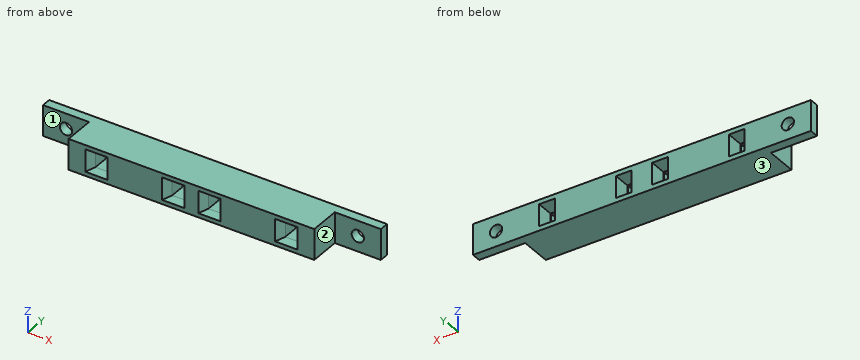
```python
from build123d import *

# Parameters (mm, degrees)
SKETCH1_W           = 80
SKETCH1_H           = 10
BOSS_EXTRUDE1_DEPTH = 10
SKETCH2_W           = 4.7
SKETCH2_H           = 6.7
CUT_EXTRUDE1_DEPTH  = 7
SKETCH3_W           = 4.7
SKETCH3_H           = 6.7
SKETCH4_W           = 7.3
SKETCH4_H           = 7.3
SKETCH5_W           = 4.7
SKETCH5_H           = 6.7
SKETCH6_W           = 7.3
SKETCH6_H           = 7.3
SKETCH8_W           = 4.7
SKETCH8_H           = 6.7
SKETCH9_W           = 7.3
SKETCH9_H           = 7.3
SKETCH10_W          = 4.7
SKETCH10_H          = 6.7
SKETCH11_W          = 7.3
SKETCH11_H          = 7.3
SKETCH12_W          = 110
SKETCH12_H          = 10
SKETCH12_W_2        = 4.7
SKETCH12_H_2        = 6.7
BOSS_EXTRUDE2_DEPTH = 3
SKETCH13_W          = 5.1
SKETCH13_H          = 7.1
CUT_EXTRUDE2_DEPTH  = 5.5
SKETCH14_R          = 2
CUT_EXTRUDE3_DEPTH  = 10


with BuildPart() as part:
    # Sketch1 → Boss-Extrude1 (new body)
    with BuildSketch(Plane(origin=(0, 0, 0), x_dir=(1, 0, 0), z_dir=(0, 1, 0))):
        with Locations((-32.862980486, 9.613188287)):
            Rectangle(SKETCH1_W, SKETCH1_H)
    extrude(amount=BOSS_EXTRUDE1_DEPTH)

    # Sketch2 → Cut-Extrude1 (cut)
    with BuildSketch(Plane(origin=(0, 10, 0), x_dir=(1, 0, 0), z_dir=(0, 1, 0))):
        with Locations((-26.962980486, 9.613188287)):
            Rectangle(SKETCH2_W, SKETCH2_H)
        with Locations((-38.762980486, 9.613188287)):
            Rectangle(SKETCH2_W, SKETCH2_H)
        with Locations((-1.962980486, 9.613188287)):
            Rectangle(SKETCH2_W, SKETCH2_H)
        with Locations((-63.762980486, 9.613188287)):
            Rectangle(SKETCH2_W, SKETCH2_H)
    extrude(amount=-CUT_EXTRUDE1_DEPTH, mode=Mode.SUBTRACT)

    # Sketch3 → Cut-Loft1 section 0
    with BuildSketch(Plane(origin=(0, 3, 0), x_dir=(1, 0, 0), z_dir=(0, 1, 0))):
        with Locations((-38.762980486, 9.613188287)):
            Rectangle(SKETCH3_W, SKETCH3_H)
    # Sketch4 → Cut-Loft1 section 1
    with BuildSketch(Plane.XZ):
        with Locations((-38.762980486, -9.613188287)):
            Rectangle(SKETCH4_W, SKETCH4_H)
    loft(mode=Mode.SUBTRACT)

    # Sketch5 → Cut-Loft2 section 0
    with BuildSketch(Plane(origin=(0, 3, 0), x_dir=(1, 0, 0), z_dir=(0, 1, 0))):
        with Locations((-63.762980486, 9.613188287)):
            Rectangle(SKETCH5_W, SKETCH5_H)
    # Sketch6 → Cut-Loft2 section 1
    with BuildSketch(Plane.XZ):
        with Locations((-63.762980486, -9.613188287)):
            Rectangle(SKETCH6_W, SKETCH6_H)
    loft(mode=Mode.SUBTRACT)

    # Sketch8 → Cut-Loft3 section 0
    with BuildSketch(Plane(origin=(0, 3, 0), x_dir=(1, 0, 0), z_dir=(0, 1, 0))):
        with Locations((-26.962980486, 9.613188287)):
            Rectangle(SKETCH8_W, SKETCH8_H)
    # Sketch9 → Cut-Loft3 section 1
    with BuildSketch(Plane.XZ):
        with Locations((-26.962980486, -9.613188287)):
            Rectangle(SKETCH9_W, SKETCH9_H)
    loft(mode=Mode.SUBTRACT)

    # Sketch10 → Cut-Loft4 section 0
    with BuildSketch(Plane(origin=(0, 3, 0), x_dir=(1, 0, 0), z_dir=(0, 1, 0))):
        with Locations((-1.962980486, 9.613188287)):
            Rectangle(SKETCH10_W, SKETCH10_H)
    # Sketch11 → Cut-Loft4 section 1
    with BuildSketch(Plane.XZ):
        with Locations((-1.962980486, -9.613188287)):
            Rectangle(SKETCH11_W, SKETCH11_H)
    loft(mode=Mode.SUBTRACT)

    # Sketch12 → Boss-Extrude2 (add)
    with BuildSketch(Plane(origin=(0, 10, 0), x_dir=(1, 0, 0), z_dir=(0, 1, 0))):
        with Locations((-32.862980486, 9.613188287)):
            Rectangle(SKETCH12_W, SKETCH12_H)
        with Locations((-63.762980486, 9.613188287)):
            Rectangle(SKETCH12_W_2, SKETCH12_H_2, mode=Mode.SUBTRACT)
        with Locations((-38.762980486, 9.613188287)):
            Rectangle(SKETCH12_W_2, SKETCH12_H_2, mode=Mode.SUBTRACT)
        with Locations((-26.962980486, 9.613188287)):
            Rectangle(SKETCH12_W_2, SKETCH12_H_2, mode=Mode.SUBTRACT)
        with Locations((-1.962980486, 9.613188287)):
            Rectangle(SKETCH12_W_2, SKETCH12_H_2, mode=Mode.SUBTRACT)
    extrude(amount=BOSS_EXTRUDE2_DEPTH)

    # Sketch13 → Cut-Extrude2 (cut)
    with BuildSketch(Plane(origin=(0, 13, 0), x_dir=(1, 0, 0), z_dir=(0, 1, 0))):
        with Locations((-63.762980486, 9.613188287)):
            Rectangle(SKETCH13_W, SKETCH13_H)
        with Locations((-38.762980486, 9.613188287)):
            Rectangle(SKETCH13_W, SKETCH13_H)
        with Locations((-26.962980486, 9.613188287)):
            Rectangle(SKETCH13_W, SKETCH13_H)
        with Locations((-1.962980486, 9.613188287)):
            Rectangle(SKETCH13_W, SKETCH13_H)
    extrude(amount=-CUT_EXTRUDE2_DEPTH, mode=Mode.SUBTRACT)

    # Sketch14 → Cut-Extrude3 (cut)
    with BuildSketch(Plane(origin=(0, 13, 0), x_dir=(1, 0, 0), z_dir=(0, 1, 0))):
        with Locations((14.637019514, 9.613188287)):
            Circle(SKETCH14_R)
        with Locations((-80.362980486, 9.613188287)):
            Circle(SKETCH14_R)
    extrude(amount=-CUT_EXTRUDE3_DEPTH, mode=Mode.SUBTRACT)


solid = part.part
```
Geometry check sheet. Reference: the model listing, model coordinates, mm. Face numbers are marked on the shaded views. A direction names the side the tool comes from. Coordinates: 2 decimals unless noted, no trailing zeros. Loops run counter-clockwise (first coordinate to the right, second up) from the corner with the lowest first, then second, coordinate; pieces in that order, holes last.
Item 1: Sectioned sample at B-B, the plane x = 15.5. Record the boundary of the cut face in (y, z), then the cut area to 3 significant figures.
Item 2: Go/stop test with flat-tipped pins: pin 1 Ø1.6 at (y, z) = (9, -11.5) entering from -X; pin 2 Ø2 at (y, z) = (8, -11) entering from +X; pin 3 Ø6 at (x, z) = (-57.5, -9) entering from -Y; pin 4 Ø5 at (x, z) = (-80.36, -9.61) entering from -Y. Record where each tip stops, or that it passes through.
Item 3: Thickness scan on line 1 (X direction, y = 3, z = -7); line 2 (X direction, y = 8.25, z = -8.75); line 3 (Z direction, x = -64.5, y = 11.25). Record the ranges inside material, lowest first.
Item 4: Sectioned sample at A-A, the plane y = 4.5. Record the boundary of the cut face in (x, z).
Item 5: Access from +Z, -Z, +X, -X, +Y, -Y to the whole of each face (thin tool, end or side, straight path). Record for the marked faces 1, 2 and 3.
Item 6: Sectioned sample at C-C, the plane y = 8.5. Record the boundary of the cut face in (x, z), then the cut area to 3 significant figures.
Check result:
1. outline: (10, -14.61) - (13, -14.61) - (13, -11.42) - (10, -11.42) - close; (10, -7.81) - (13, -7.81) - (13, -4.61) - (10, -4.61) - close
1. area: 19.2 mm2
2. pin 1: stops at x = -72.86
2. pin 2: stops at x = 7.14
2. pin 3: stops at y = 0
2. pin 4: stops at y = 10
3. line 1: x = -72.86 to -66.11, -61.41 to -41.11, -36.41 to -29.31, -24.61 to -4.31, 0.39 to 7.14
3. line 2: x = -72.86 to -66.31, -61.21 to -41.31, -36.21 to -29.51, -24.41 to -4.51, 0.59 to 7.14
3. line 3: z = -14.61 to -13.16, -6.06 to -4.61
4. outline: (-72.86, -14.61) - (7.14, -14.61) - (7.14, -4.61) - (-72.86, -4.61) - close; hole (-66.11, -12.96) - (-61.41, -12.96) - (-61.41, -6.26) - (-66.11, -6.26) - close; hole (-41.11, -12.96) - (-36.41, -12.96) - (-36.41, -6.26) - (-41.11, -6.26) - close; hole (-29.31, -12.96) - (-24.61, -12.96) - (-24.61, -6.26) - (-29.31, -6.26) - close; hole (-4.31, -12.96) - (0.39, -12.96) - (0.39, -6.26) - (-4.31, -6.26) - close
5. face 1: +Z, -Z, -X, -Y
5. face 2: +Z, -Z, +X, -Y
5. face 3: -Z, +X, -X, +Y, -Y
6. outline: (-72.86, -14.61) - (7.14, -14.61) - (7.14, -4.61) - (-72.86, -4.61) - close; hole (-66.31, -13.16) - (-61.21, -13.16) - (-61.21, -6.06) - (-66.31, -6.06) - close; hole (-41.31, -13.16) - (-36.21, -13.16) - (-36.21, -6.06) - (-41.31, -6.06) - close; hole (-29.51, -13.16) - (-24.41, -13.16) - (-24.41, -6.06) - (-29.51, -6.06) - close; hole (-4.51, -13.16) - (0.59, -13.16) - (0.59, -6.06) - (-4.51, -6.06) - close
6. area: 655 mm2
